Verification items for the finished model (mm, model axes). A direction names the side the tool comes from. Coordinates: 2 decimals unless noted, no trailing zeros. Order: outer loops, then holes, each group sorted by start corner. A loop starts at its lowest first (then second) coordinate and runs counter-clockwise, first axis right, second up. Notation, with made-up numbers: M 74.5,0 L 93.5,0 A21 cw 93.5,39 Z; hole C 31,48.5 d11. An arc over 180 degrees is marked long. Return JSON: item names as keys, results as strings.
Autodesk Inventor part; units mm, degrees
ref_plane "YZ Plane" through (0, 0, 0) normal (1, 0, 0) x (0, 1, 0)
ref_plane "XZ Plane" through (0, 0, 0) normal (0, 1, 0) x (-1, 0, 0)
ref_plane "XY Plane" through (0, 0, 0) normal (0, 0, 1) x (1, 0, 0)
sketch "Sketch1" plane through (0, 0, 0) normal (0, 1, 0) x (-1, 0, 0)
  line L0 (23.5265, 54.5795) -> (-113.4735, 54.5795)
  line L1 (-113.4735, 54.5795) -> (-113.4735, -435.4205)
  line L2 (-113.4735, -435.4205) -> (23.5265, -435.4205)
  line L3 (23.5265, -435.4205) -> (23.5265, 54.5795)
  point P0 (0, 0)
  dimension "d0" = 137
  dimension "d1" = 490
extrude "Extrusion1" add sketch "Sketch1" along normal blind 15
sketch "Sketch2" plane through (-23.5265, 0, 54.5795) normal (0, 0, 1) x (1, 0, 0)
  line L0 (137, 0) -> (0, 0)
  line L1 (0, 0) -> (127, 0)
  line L2 (127, 0) -> (127, 5)
  line L3 (127, 5) -> (0, 5)
  line L4 (0, 5) -> (0, 0)
  point P0 (23.5265, 0)
  dimension "d4" = 127
  dimension "d5" = 5
extrude "Extrusion2" cut sketch "Sketch2" against normal blind 7
sketch "Sketch3" plane through (113.4735, 0, -435.4205) normal (0, 0, -1) x (-1, 0, 0)
  line L0 (0, 0) -> (137, 0)
  line L1 (0, 0) -> (137, 0)
  line L2 (137, 0) -> (137, 5)
  line L3 (137, 5) -> (0, 5)
  line L4 (0, 5) -> (0, 0)
  point P0 (113.4735, 0)
  dimension "d8" = 137
  dimension "d9" = 5
extrude "Extrusion3" cut sketch "Sketch3" against normal blind 7
sketch "Sketch4" plane through (0, 0, 0) normal (0, -1, 0) x (1, 0, 0)
  line L0 (-23.5265, -428.4205) -> (113.4735, -428.4205)
  line L1 (103.4735, 47.5795) -> (-23.5265, 47.5795)
  line L2 (113.4735, -428.4205) -> (103.4735, -428.4205)
  line L3 (103.4735, -428.4205) -> (103.4735, 47.5795)
  line L4 (103.4735, 47.5795) -> (113.4735, 47.5795)
  line L5 (113.4735, 47.5795) -> (113.4735, -428.4205)
  point P0 (0, 0)
  point P1 (-13.5265, -428.4205)
  dimension "d12" = 10
  dimension "d13" = 476
extrude "Extrusion4" cut sketch "Sketch4" against normal blind 5
sketch "Sketch5" plane through (0, 15, 0) normal (0, 1, 0) x (1, 0, 0)
  circle A0 centre (22.1402, 68.4205) radius 15
  circle A1 centre (67.8068, 128.4205) radius 15
  circle A2 centre (44.9735, 228.4205) radius 20
  line L0 (103.4735, 428.4205) -> (-23.5265, 428.4205)
  line L1 (-23.5265, 435.4205) -> (-23.5265, -54.5795)
  point P0 (0, 0)
  point P1 (-13.5265, 428.4205)
  dimension "d16" = 40
  dimension "d17" = 200
  dimension "d18" = 68.5
  dimension "d19" = 300
  dimension "d20" = 91.3333
  dimension "d21" = 45.6667
  dimension "d22" = 360
  dimension "d23" = 30
  dimension "d24" = 30
extrude "Extrusion5" cut sketch "Sketch5" against normal blind 15
sketch "Sketch6" plane through (0, 0, 0) normal (0, -1, 0) x (1, 0, 0)
  line L0 (69.9735, -253.4205) -> (19.9735, -253.4205)
  line L1 (19.9735, -253.4205) -> (19.9735, -203.4205)
  line L2 (19.9735, -203.4205) -> (69.9735, -203.4205)
  line L3 (69.9735, -203.4205) -> (69.9735, -253.4205)
  circle A0 centre (44.9735, -228.4205) radius 20
  point P0 (0, 0)
  dimension "d27" = 25
  dimension "d28" = 50
  dimension "d29" = 25
  dimension "d30" = 50
extrude "Extrusion6" cut sketch "Sketch6" against normal blind 12
sketch "Sketch7" plane through (0, 15, 0) normal (0, 1, 0) x (1, 0, 0)
  circle A0 centre (44.9735, 228.4205) radius 20
  point P0 (0, 0)
  point P1 (28.7235, 212.1705)
  point P2 (28.7235, 244.6705)
  point P3 (61.2235, 244.6705)
  point P4 (61.2235, 212.1705)
  dimension "d33" = 16.25
  dimension "d34" = 16.25
  dimension "d35" = 16.25
  dimension "d36" = 16.25
  dimension "d37" = 16.25
  dimension "d38" = 16.25
  dimension "d39" = 16.25
  dimension "d40" = 16.25
hole "Hole1" at (28.7235, 15, -212.1705) at (28.7235, 15, -244.6705) at (61.2235, 15, -244.6705) at (61.2235, 15, -212.1705) direction (0, -1, 0) diameter 2.5 end through all
sketch "Sketch8" plane through (0, 0, 0) normal (0, -1, 0) x (1, 0, 0)
  circle A0 centre (61.2235, -244.6705) radius 1.25
  circle A1 centre (28.7235, -212.1705) radius 1.25
  circle A2 centre (28.7235, -244.6705) radius 1.25
  circle A3 centre (61.2235, -212.1705) radius 1.25
  line L0 (19.9735, -203.4205) -> (69.9735, -203.4205)
  line L1 (19.9735, -253.4205) -> (19.9735, -203.4205)
  line L2 (69.9735, -253.4205) -> (19.9735, -253.4205)
  line L3 (69.9735, -203.4205) -> (69.9735, -253.4205)
  circle A4 centre (44.9735, -228.4205) radius 20
  line L4 (69.9735, -203.4205) -> (69.9735, -253.4205)
  line L5 (69.9735, -253.4205) -> (79.9735, -253.4205)
  line L6 (79.9735, -253.4205) -> (79.9735, -203.4205)
  line L7 (79.9735, -203.4205) -> (69.9735, -203.4205)
  line L8 (69.9735, -203.4205) -> (69.9735, -253.4205)
  line L9 (79.9735, -203.4205) -> (19.9735, -203.4205)
  line L10 (19.9735, -203.4205) -> (19.9735, -193.4205)
  line L11 (19.9735, -193.4205) -> (79.9735, -193.4205)
  line L12 (79.9735, -193.4205) -> (79.9735, -203.4205)
  point P0 (0, 0)
  dimension "d48" = 10
  dimension "d49" = 50
  dimension "d50" = 60
  dimension "d51" = 10
extrude "Extrusion7" cut sketch "Sketch8" against normal blind 12 contours L10 L11 L12 L7 L0 | L7 L6 L5 L3
sketch "Sketch9" plane through (0, 15, 0) normal (0, 1, 0) x (1, 0, 0)
  line L0 (43.4735, 338.4205) -> (83.4735, 338.4205)
  line L1 (83.4735, 338.4205) -> (83.4735, 398.4205)
  line L2 (83.4735, 398.4205) -> (43.4735, 398.4205)
  line L3 (43.4735, 398.4205) -> (43.4735, 338.4205)
  line L4 (103.4735, 428.4205) -> (-23.5265, 428.4205)
  line L5 (113.4735, -54.5795) -> (113.4735, 435.4205)
  line L6 (46.6735, 342.9072) -> (52.6735, 342.9072)
  line L7 (52.6735, 342.9072) -> (52.6735, 392.9072)
  line L8 (52.6735, 392.9072) -> (46.6735, 392.9072)
  line L9 (46.6735, 392.9072) -> (46.6735, 342.9072)
  line L10 (55.8735, 342.9072) -> (61.8735, 342.9072)
  line L11 (61.8735, 342.9072) -> (61.8735, 392.9072)
  line L12 (61.8735, 392.9072) -> (55.8735, 392.9072)
  line L13 (55.8735, 392.9072) -> (55.8735, 342.9072)
  line L14 (65.0735, 342.9072) -> (71.0735, 342.9072)
  line L15 (71.0735, 342.9072) -> (71.0735, 392.9072)
  line L16 (71.0735, 392.9072) -> (65.0735, 392.9072)
  line L17 (65.0735, 392.9072) -> (65.0735, 342.9072)
  line L18 (74.2735, 342.9072) -> (80.2735, 342.9072)
  line L19 (80.2735, 342.9072) -> (80.2735, 392.9072)
  line L20 (80.2735, 392.9072) -> (74.2735, 392.9072)
  line L21 (74.2735, 392.9072) -> (74.2735, 342.9072)
  point P0 (0, 0)
  point P1 (-13.5265, 428.4205)
  dimension "d54" = 60
  dimension "d55" = 40
  dimension "d56" = 30
  dimension "d57" = 30
  dimension "d58" = 50
  dimension "d59" = 50
  dimension "d60" = 6
  dimension "d61" = 6
  dimension "d62" = 6
  dimension "d63" = 6
  dimension "d64" = 3.2
  dimension "d65" = 3.2
  dimension "d66" = 3.2
  dimension "d67" = 3.2
extrude "Extrusion8" cut sketch "Sketch9" against normal blind 15 contours L9 L8 L7 L6 | L13 L12 L11 L10 | L17 L16 L15 L14 | L21 L20 L19 L18
sketch "Sketch11" plane through (0, 0, 0) normal (0, -1, 0) x (1, 0, 0)
  line L0 (103.4735, -400.4205) -> (23.4735, -400.4205)
  line L1 (23.4735, -400.4205) -> (23.4735, -285.4205)
  line L2 (23.4735, -285.4205) -> (103.4735, -285.4205)
  line L3 (103.4735, -285.4205) -> (103.4735, -400.4205)
  line L4 (113.4735, 47.5795) -> (113.4735, -435.4205)
  line L5 (113.4735, -435.4205) -> (-23.5265, -435.4205)
  point P0 (0, 0)
  point P1 (-13.5265, -435.4205)
  dimension "d70" = 80
  dimension "d71" = 115
  dimension "d72" = 10
  dimension "d73" = 35
extrude "Extrusion9" cut sketch "Sketch11" against normal blind 10
sketch "Sketch12" plane through (-23.5265, 15, 54.5795) normal (0, 0, 1) x (1, 0, 0)
  line L0 (0, 0) -> (137, 0)
  line L1 (137, -121) -> (137, 0)
  line L2 (127, -15) -> (137, -15)
  line L3 (127, -10) -> (127, -121)
  line L4 (0, -10) -> (127, -10)
  line L5 (127, -10) -> (127, -121)
  line L6 (0, -10) -> (127, -10)
  line L7 (137, -15) -> (137, -10)
  line L8 (127, -10) -> (137, -10)
  line L9 (137, -10) -> (137, -15)
  line L10 (137, -15) -> (127, -15)
  line L11 (127, -15) -> (127, -10)
  point P0 (23.5265, -15)
extrude "Extrusion10" cut sketch "Sketch12" against normal blind 7
properties part number "Arcade_ControlTop"
Q1. Go/stop test with flat-tipped pins: pin 1 (2 mm diameter, centred on x = 61.22, z = -244.67, fed in from +Y); pin 2 (3 mm diameter, centred on x = 97, z = -265, fed in from -Y); pin 3 (4 mm diameter, centred on x = 67, y = 1.5, fed in from +Z). Record where each tip stops, or that it passes through.
Values:
{"pin 1": "through", "pin 2": "y = 0", "pin 3": "z = 47.58"}
Q2. Tool access check on faces 5 (the face through (50, 6, -253.42)), 6 (the face through (65.9, 7.6, -143.3)). Record the directions out of +Z, -Z, +X, -X, +Y, -Y that give a thin tool (end or side, any length) a straight path to the whole face; none if there is none.
Values:
{"face 5": "-Y", "face 6": "+Y, -Y"}
Q3. Cross-section at A-A, the plane z = -366. Record the boundary of the cut face in (x, y), and give its area (4 significant figures).
Values:
{"outline": "M -23.53,0 L 23.47,0 L 23.47,10 L 46.67,10 L 46.67,15 L -23.53,15 Z; M 52.67,10 L 55.87,10 L 55.87,15 L 52.67,15 Z; M 61.87,10 L 65.07,10 L 65.07,15 L 61.87,15 Z; M 71.07,10 L 74.27,10 L 74.27,15 L 71.07,15 Z; M 80.27,10 L 103.47,10 L 103.47,5 L 113.47,5 L 113.47,15 L 80.27,15 Z", "area": "1,085 mm^2"}
Q4. Cross-section at C-C, the plane z = -122.5. Record the boundary of the cut face in (x, y), and give its area (3 significant figures).
Values:
{"outline": "M -23.53,0 L 54.02,0 L 54.02,15 L -23.53,15 Z; M 81.59,0 L 103.47,0 L 103.47,5 L 113.47,5 L 113.47,15 L 81.59,15 Z", "area": "1,590 mm^2"}
Q5. Cross-section at B-B, the plane z = -309. Record the boundary of the cut face in (x, y).
Values:
{"outline": "M -23.53,0 L 23.47,0 L 23.47,10 L 103.47,10 L 103.47,5 L 113.47,5 L 113.47,15 L -23.53,15 Z"}
Q6. Draft check along X on faces 1 (the face through (113.474, 10, -187)), 2 (the face through (46, 15, -187)), 3 (the face through (-23.526, 7, -194)), 4 (the face through (63, 5, -285.42)). Enter one of: pulls with the +X half, pulls with the -X half, needs draft (parallel to the pull), parting line crosses it, or undercut.
Values:
{"face 1": "pulls with the +X half", "face 2": "needs draft", "face 3": "pulls with the -X half", "face 4": "undercut"}
Q7. Material ranges on line 1 along Z through (x, y) = (21, 1.25); line 2 along Z through (x, y) = (21.5, 10); line 3 along X through (y, z) = (9.25, -337.5), recorded low to high.
Values:
{"line 1": "-428.42 to -253.42, -193.42 to -83.38, -53.46 to 47.58", "line 2": "-435.42 to -253.42, -193.42 to -83.41, -53.43 to 54.58", "line 3": "-23.53 to 23.47, 103.47 to 113.47"}
